Build history of the part. All positions in model axes, mm. Face numbers are marked on the shaded views. A direction names the side the tool comes from. Round coordinates to 2 decimals unless told otherwise and drop trailing zeros. Order: outer loops, then holes, each group sorted by start corner. A loop starts at its lowest first (then second) coordinate and runs counter-clockwise, first axis right, second up. Notation, with made-up numbers: M 31.5,70 L 40.5,70 A12 cw 40.5,78 Z; hole C -17,47.25 d10. An arc over 180 degrees is marked long. One line per item, written item: value. Start each with the question number.
Item 1: Band-saw the part on A-A, the plane z = 22.5. Write the cut outline in (x, y).
Item 2: Tool access for the marked faces 5 and 6: list every direction of +Z, -Z, +X, -X, +Y, -Y with a clear straight run to the whole face (end or side of a thin tool).
Item 3: Band-saw the part on D-D, the plane x = 21. Write the cut outline in (y, z), then the cut area to 3 significant figures.
Item 4: Two-plate mould, pull along Y, no slides. Class the marked faces 1, 2, 3 and 4: +Y half, -Y half, draft (parallel to the pull), parting line (faces both ways), or undercut.
Item 5: Pin check, flat tips, straight feed: pin 1 (4.5 mm diameter, centred on x = -4.44, y = 28.79, fed in from +Z) (3 decimals); pin 2 (3 mm diameter, centred on y = -4.5, z = 14.5, fed in from +X); pin 3 (10 mm diameter, centred on x = 4.44, y = 28.79, fed in from +Z); pin 4 (10 mm diameter, centred on y = 35.5, z = 14.5, fed in from -X). Stop position of each tip, or through.
Item 6: Band-saw the part on C-C, the plane y = 26.5. Write the cut outline in (x, z).
Item 7: Probe L1, parallel to Z at x = -4.5, y = -24.5; L2, parallel to X at y = -9, z = 40.5; L3, parallel to Y at x = -13, z = 4.5. List the from-to ranges inside material, lowest first.
Item 8: Band-saw the part on B-B, the plane x = -3.5. Write the cut outline in (y, z), then the cut area to 3 significant figures.
```python
from build123d import *

# Parameters (mm, degrees)
F1_DEPTH = 50.8
F2_T     = -2.54
F3_R     = 3.81
F4_DEPTH = 25.4


with BuildPart() as f1:
    # F0 (on Top) → F1 (new body)
    with BuildSketch(Plane.XY):
        Polygon((0, -55.765115), (0, 20.321534), (-38.1, 20.321534), (-19.05, -55.765115), align=None)
        Polygon((38.1, 20.321534), (0, 20.321534), (0, -55.765115), (19.05, -55.765115), align=None)
        Polygon((38.1, 20.321534), (0, 71.121534), (0, 20.321534), align=None)
        Polygon((0, 20.321534), (0, 71.121534), (-38.1, 20.321534), align=None)
    extrude(amount=F1_DEPTH)

    # F2
    f2_openings = [f1.faces().sort_by_distance(p)[0] for p in [
        (0, 2.136611, 50.8),
    ]]
    offset(amount=F2_T, openings=f2_openings)

    # F3 (on face) → F4 (cut)
    with BuildSketch(Plane.XY.offset(2.54)):
        with Locations((4.445, 28.7882)):
            Circle(F3_R)
        with Locations((-4.445, 28.7882)):
            Circle(F3_R)
    extrude(amount=-F4_DEPTH, mode=Mode.SUBTRACT)


solid = f1.part
```
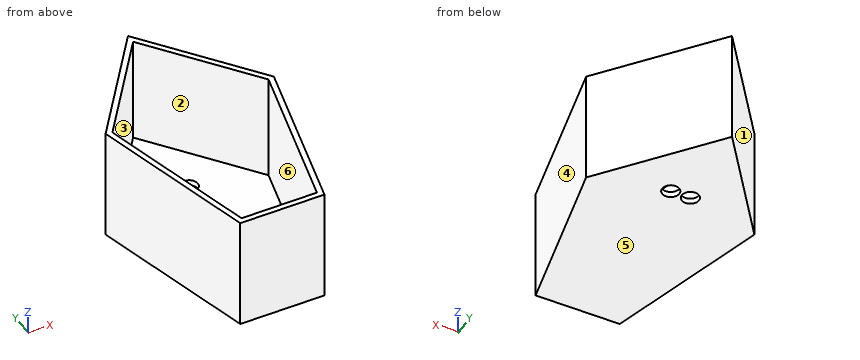
Output:
1. outline: M -38.1,20.32 L -19.05,-55.77 L 19.05,-55.77 L 38.1,20.32 L 0,71.12 Z; hole M -35.34,19.77 L -17.07,-53.23 L 17.07,-53.23 L 35.34,19.77 L 0,66.89 Z
2. face 5: -Z, +X, -X, +Y, -Y
2. face 6: +Z
3. outline: M -47.98,0 L 43.12,0 L 43.12,50.8 L 38.89,50.8 L 38.89,2.54 L -37.52,2.54 L -37.52,50.8 L -47.98,50.8 Z
3. area: 940 mm²
4. face 1: +Y half
4. face 2: undercut
4. face 3: undercut
4. face 4: -Y half
5. pin 1: passes through
5. pin 2: stops at x = 32.26
5. pin 3: stops at z = 2.54
5. pin 4: stops at x = -30.47
6. outline: M -33.47,0 L -7.49,0 L -7.49,2.54 L -30.29,2.54 L -30.29,50.8 L -33.47,50.8 Z; M -1.4,0 L 1.4,0 L 1.4,2.54 L -1.4,2.54 Z; M 7.49,0 L 33.47,0 L 33.47,50.8 L 30.29,50.8 L 30.29,2.54 L 7.49,2.54 Z
7. L1: z = 0 to 2.54
7. L2: x = -30.76 to -28.14, 28.14 to 30.76
7. L3: y = -55.77 to -53.23, 49.55 to 53.79
8. outline: M -55.77,0 L 25.1,0 L 25.1,2.54 L -53.23,2.54 L -53.23,50.8 L -55.77,50.8 Z; M 32.48,0 L 66.45,0 L 66.45,50.8 L 62.22,50.8 L 62.22,2.54 L 32.48,2.54 Z
8. area: 619 mm²
